Read the model definition and answer for the solid it produces. Units are mm, in the model's axes. A direction names the side the tool comes from. Round coordinates to 2 decimals unless told otherwise and drop trailing zeros. Loops run counter-clockwise (first coordinate to the right, second up) from the corner with the lowest first, then second, coordinate; pieces in that order, holes last. Notation, with made-up numbers: (-29.75, 80.5) - (-5.75, 80.5) arc R23 ccw to (-5.75, 112.5) - close; hole circle Ø9 at (55.5, 70.25). An arc over 180 degrees is marked (long way). Answer as CSV lines item,"result".
```python
from build123d import *

# Parameters (mm, degrees)
SKETCH1_R           = 1.5
BOSS_EXTRUDE1_DEPTH = 50
FILLET2_R           = 0.2
SKETCH2_R           = 2
BOSS_EXTRUDE2_DEPTH = 3
SKETCH3_R           = 0.5
BOSS_EXTRUDE3_DEPTH = 15


with BuildPart() as part:
    # Sketch1 → Boss-Extrude1 (new body)
    with BuildSketch(Plane.XY):
        Circle(SKETCH1_R)
    extrude(amount=BOSS_EXTRUDE1_DEPTH)

    # Fillet2
    fillet2_edges = [part.edges().sort_by_distance(p)[0] for p in [
        (-1.5, 0, 50),
    ]]
    fillet(fillet2_edges, radius=FILLET2_R)

    # Sketch2 → Boss-Extrude2 (add)
    with BuildSketch(Plane(origin=(0, 0, 0), x_dir=(-1, 0, 0), z_dir=(0, 0, -1))):
        Circle(SKETCH2_R)
    extrude(amount=BOSS_EXTRUDE2_DEPTH)

    # Sketch3 → Boss-Extrude3 (add)
    with BuildSketch(Plane(origin=(0, 0, -3), x_dir=(-1, 0, 0), z_dir=(0, 0, -1))):
        Circle(SKETCH3_R)
    extrude(amount=BOSS_EXTRUDE3_DEPTH)


solid = part.part
```
1) A tool of negligible diameter and unlimited length cuts with its end or side. For faces 1 (the face through (0.5, 0.5, -3)), 2 (the face through (-1.5, 0.07, 24.55)), 3 (the face through (0, -2, -1)), from which of +Z, -Z, +X, -X, +Y, -Y can it reach the whole face along a straight path? Write none if from no direction.
Entries:
face 1,"-Z"
face 2,"+Z"
face 3,"+Z, -Z"
2) Find the intervals of material crossed by line 1 (Y direction, x = 0.15, z = -0.5); line 2 (Z direction, x = 1.85, y = 0.2); line 3 (Z direction, x = 0.7, y = -0.2), in increasing order.
Entries:
line 1,"y = -1.99 to 1.99"
line 2,"z = -3 to 0"
line 3,"z = -3 to 50"
3) A cutting plane is placed at A-A, the plane z = 35. Determine the outline of the cut face in (x, y).
Entries:
outline,"circle Ø3 at (0, 0)"
